Part print with two shaded views. Sizes in mm from the minimum x, y, z corner. Coordinates: 2 decimals unless noted, no trailing zeros. Loops run counter-clockwise (first coordinate to the right, second up) from the corner with the lowest first, then second, coordinate; pieces in that order, holes last.
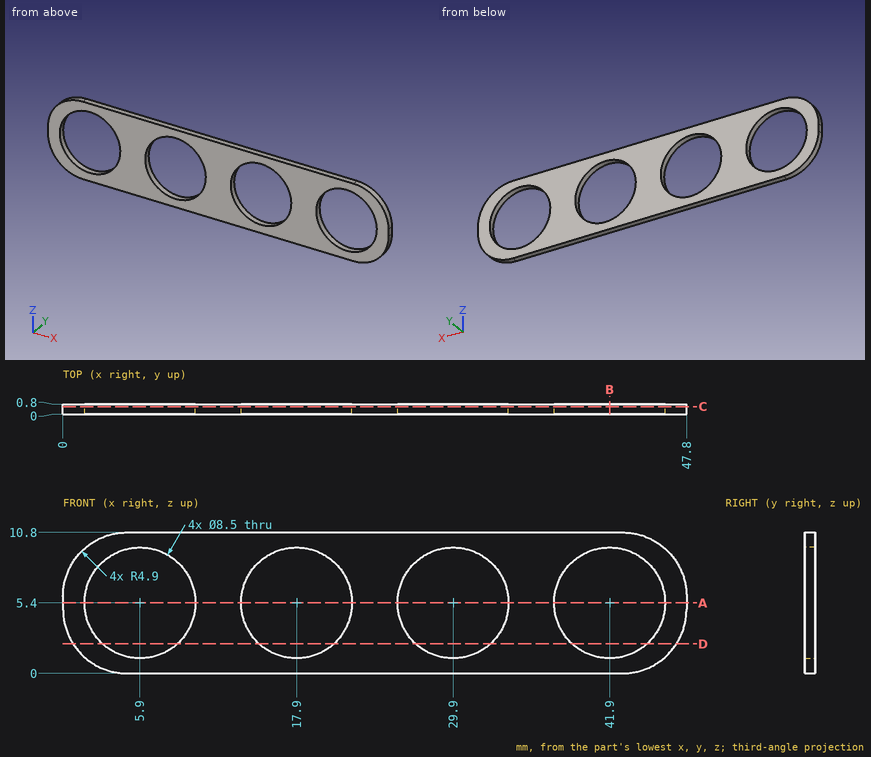
Q1. Slice it at A-A (z = 5.4). List the corners of the cut face in (x, y), and give its area (3 significant figures).
Answers:
outline: (0, 0) - (1.65, 0) - (1.65, 0.8) - (0, 0.8) - close; (10.15, 0) - (13.65, 0) - (13.65, 0.8) - (10.15, 0.8) - close; (22.15, 0) - (25.65, 0) - (25.65, 0.8) - (22.15, 0.8) - close; (34.15, 0) - (37.65, 0) - (37.65, 0.8) - (34.15, 0.8) - close; (46.15, 0) - (47.8, 0) - (47.8, 0.8) - (46.15, 0.8) - close
area: 11.0 mm2
Q2. Drill centre lines: line 1 (X direction, y = 0.65, z = 5.4); line 2 (X direction, y = 0.65, z = 7.25); line 3 (Z direction, x = 17, y = 0.15). Where is each one in solid material? Low to high.
Answers:
line 1: x = 0 to 1.65, 10.15 to 13.65, 22.15 to 25.65, 34.15 to 37.65, 46.15 to 47.8
line 2: x = 0.19 to 2.07, 9.73 to 14.07, 21.73 to 26.07, 33.73 to 38.07, 45.73 to 47.61
line 3: z = 0 to 1.25, 9.55 to 10.8
Q3. Slice it at C-C (y = 0.6). List the corners of the cut face in (x, z).
Answers:
outline: (0, 4.9) arc R4.9 ccw to (4.9, 0) - (42.9, 0) arc R4.9 ccw to (47.8, 4.9) - (47.8, 5.9) arc R4.9 ccw to (42.9, 10.8) - (4.9, 10.8) arc R4.9 ccw to (0, 5.9) - close; hole circle Ø8.5 at (5.9, 5.4); hole circle Ø8.5 at (17.9, 5.4); hole circle Ø8.5 at (29.9, 5.4); hole circle Ø8.5 at (41.9, 5.4)
Q4. Slice it at D-D (z = 2.25). List the corners of the cut face in (x, y).
Answers:
outline: (0.78, 0) - (3.05, 0) - (3.05, 0.8) - (0.78, 0.8) - close; (8.75, 0) - (15.05, 0) - (15.05, 0.8) - (8.75, 0.8) - close; (20.75, 0) - (27.05, 0) - (27.05, 0.8) - (20.75, 0.8) - close; (32.75, 0) - (39.05, 0) - (39.05, 0.8) - (32.75, 0.8) - close; (44.75, 0) - (47.02, 0) - (47.02, 0.8) - (44.75, 0.8) - close
Q5. Slice it at B-B (x = 41.9). List the corners of the cut face in (y, z), and give its area (3 significant figures).
Answers:
outline: (0, 0) - (0.8, 0) - (0.8, 1.15) - (0, 1.15) - close; (0, 9.65) - (0.8, 9.65) - (0.8, 10.8) - (0, 10.8) - close
area: 1.84 mm2
